Can you work these out from the drawing? Everything is in mm from the part's minimum corner. A direction names the side the tool comes from. Coordinates: 2 decimals unless noted, no trailing zeros. Order: outer loops, then holes, each group sorted by start corner. A loop starts at its lowest first (then second) coordinate and runs counter-clockwise, first axis right, second up. Notation, with made-up numbers: (-6.5, 84) -> (39.5, 84) arc R12 ccw to (39.5, 91) -> close; hole circle Ø1 at (-19.75, 82). An arc over 180 degrees is marked (long way). Return JSON: item names as keys, results as strings. Group by question number.
1) For the marked faces 5 and 6, which set-ups out of +Z, -Z, +X, -X, +Y, -Y let a thin tool reach every point of the face, with its end or its side?
2) If I drill on probe 1 along Y at (x, z) = (4, 12.5); probe 2 along Y at (x, z) = (17.75, 18.5); probe 3 along X at (y, z) = (18.75, 3.5), over which ranges is the centre line in solid material (lowest first)? Write a range as from..to.
3) For pin 1 (5 mm diameter, centred on y = 21, z = 13, fed in from -X) (3 decimals); pin 2 (12 mm diameter, centred on x = 6, z = 22, fed in from +Y); pin 3 (4 mm diameter, centred on y = 10, z = 17.5, fed in from +X); pin 4 (8 mm diameter, centred on x = 13.5, z = 10, fed in from +Y), each with a flat end and sliding along its axis, tell me the tip position at first contact or that it passes through.
4) If we section it at D-D, the plane z = 17.5: Please give me the cut outline in (x, y), then the cut area to 3 significant figures.
5) Thinking about a two-plate mould opening in Z: for the marked faces 1, 2, 3 and 4, which applies, +Z half, -Z half, draft (parallel to the pull), parting line (faces both ways), or undercut?
6) If we section it at C-C, the plane y = 19.5: Please give me the cut outline in (x, z), then the cut area to 3 significant figures.
7) If we section it at A-A, the plane z = 12.5: Please give me the cut outline in (x, y), then the cut area to 3 significant figures.
8) If we section it at B-B, the plane x = 9: Please give me the cut outline in (y, z), then the cut area to 3 significant figures.
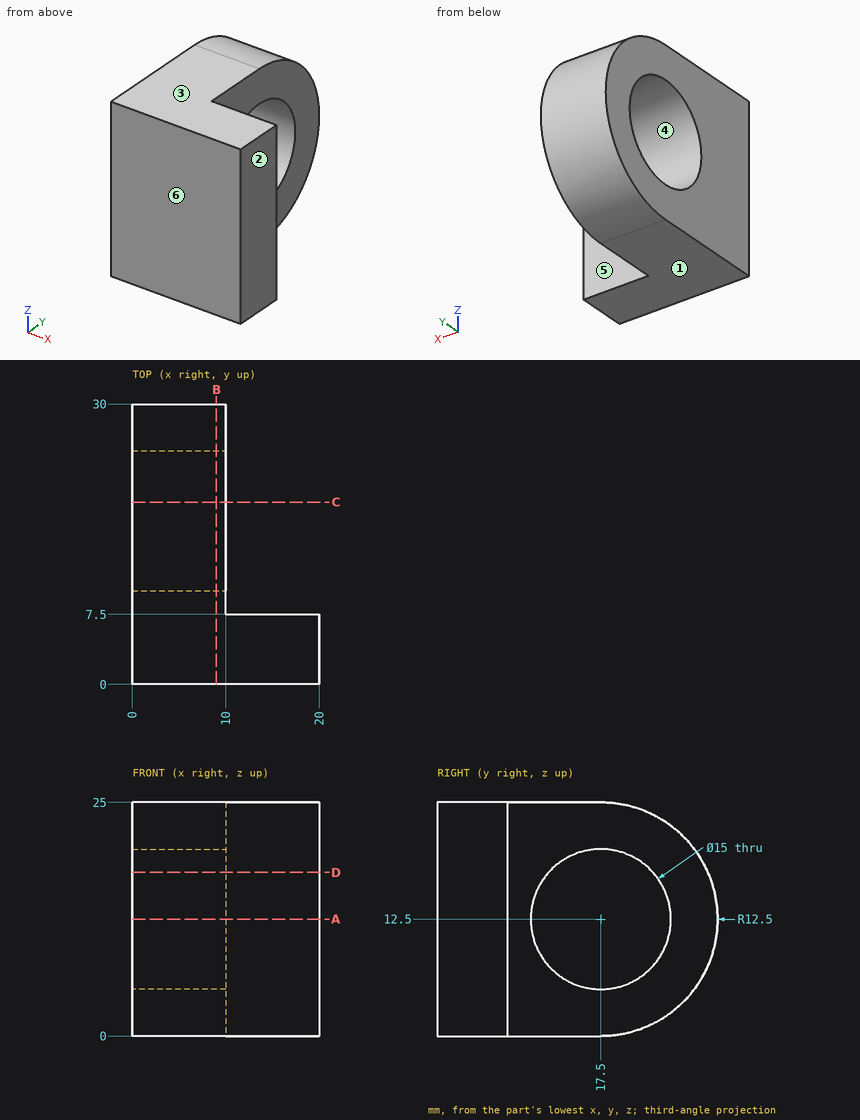
Result sheet:
{
 "1": {"face 5": "+Z, -Z, +X, +Y", "face 6": "+Z, -Z, +X, -X, -Y"},
 "2": {"probe 1": "y = 0..10, 25..30", "probe 2": "y = 0..7.5", "probe 3": "x = 0..10"},
 "3": {"pin 1": "passes through", "pin 2": "stops at y = 29.5", "pin 3": "stops at x = 10", "pin 4": "stops at y = 29.99"},
 "4": {"outline": "(0, 0) -> (20, 0) -> (20, 7.5) -> (10, 7.5) -> (10, 11.91) -> (0, 11.91) -> close; (0, 23.09) -> (10, 23.09) -> (10, 28.96) -> (0, 28.96) -> close", "area": "253 mm2"},
 "5": {"face 1": "-Z half", "face 2": "draft", "face 3": "+Z half", "face 4": "undercut"},
 "6": {"outline": "(0, 0.16) -> (10, 0.16) -> (10, 5.27) -> (0, 5.27) -> close; (0, 19.73) -> (10, 19.73) -> (10, 24.84) -> (0, 24.84) -> close", "area": "102 mm2"},
 "7": {"outline": "(0, 0) -> (20, 0) -> (20, 7.5) -> (10, 7.5) -> (10, 10) -> (0, 10) -> close; (0, 25) -> (10, 25) -> (10, 30) -> (0, 30) -> close", "area": "225 mm2"},
 "8": {"outline": "(0, 0) -> (17.5, 0) arc R12.5 ccw to (17.5, 25) -> (0, 25) -> close; hole circle Ø15 at (17.5, 12.5)", "area": "506 mm2"}
}
